Check sheet for the modelled part. Datum: model origin and axes. Units: mm. A direction names the side the tool comes from. Round coordinates to 2 decimals unless told otherwise and drop trailing zeros. Order: outer loops, then holes, each group sorted by start corner. A loop starts at its lowest first (then second) coordinate and runs counter-clockwise, first axis right, second up.
(1) Sectioned sample at B-B, the plane z = 25. Enter the section's corners in (x, y), and give its area (3 significant figures).
(2) Sectioned sample at A-A, the plane z = 10. Enter the section's corners in (x, y).
(3) Sectioned sample at C-C, the plane y = -3.5. Enter the section's corners in (x, z), and give its area (3 significant figures).
(4) Tool access check on faces 5 (the flat face through (3, -20, 2)), 6 (the flat face through (0, 6.716, 13)), 7 (the cylindrical face through (1.739, -15.325, 13.205)), 8 (the cylindrical face through (2.314, -14.176, 20.762)). Record the directions out of +Z, -Z, +X, -X, +Y, -Y that give a thin tool (end or side, any length) a straight path to the whole face; none if there is none.
(5) Depth check by flat-ended pin: pin 1 (3.5 mm diameter, centred on x = -11, y = -21.5, fed in from +Z); pin 2 (3 mm diameter, centred on x = -11, z = 14.5, fed in from -Y); pin 3 (1.4 mm diameter, centred on y = 7.5, z = 11.5, fed in from +X). Enter the tip coordinate at first touch or a pass-through.
(6) Thickness scan on probe 1 along Y at (x, z) = (11.5, 13); probe 2 along Z at (x, y) = (0.5, -11.5); probe 3 along Y at (x, z) = (23, 18.5). Record the ranges inside material, lowest first.
(7) Mould release check, pull along Y, two halves, no side actions. Record for faces 1 (the flat face through (2, -6, 2)), 2 (the flat face through (22.89, -6.12, 1.01)), 3 (the cylindrical face through (-2.361, -18.603, 8.761)), 4 (the flat face through (18, -21, 2)): released by +Y, released by -Y, zero draft, split by the parting line, or undercut.
```python
from build123d import *

# Parameters (mm, degrees)
CROQUIS1_W              = 60
CROQUIS1_H              = 30
SALIENTE_EXTRUIR1_DEPTH = 2
SALIENTE_EXTRUIR2_DEPTH = 38
SALIENTE_EXTRUIR4_DEPTH = 2
REDONDEO1_R             = 2
REDONDEO2_R             = 1
CORTAR_EXTRUIR2_DEPTH   = 2
CROQUIS7_W              = 20
CROQUIS7_H              = 20
SALIENTE_EXTRUIR5_DEPTH = 2.7
CROQUIS8_R              = 1.75
CORTAR_EXTRUIR3_DEPTH   = 2.7
CROQUIS11_R             = 3.36
CORTAR_EXTRUIR4_DEPTH   = 50
SALIENTE_EXTRUIR3_DEPTH = 15
CORTAR_EXTRUIR1_START   = -12.5
CORTAR_EXTRUIR1_DEPTH   = 12.5


with BuildPart() as part:
    # Croquis1 → Saliente-Extruir1 (new body)
    with BuildSketch(Plane.XY):
        with Locations((2.747988453, -8.28358209)):
            Rectangle(CROQUIS1_W, CROQUIS1_H)
    extrude(amount=SALIENTE_EXTRUIR1_DEPTH)

    # Croquis2 → Saliente-Extruir2 (add)
    with BuildSketch(Plane.XY.offset(2)):
        with BuildLine():
            Line((-27.252011547, -23.28358209), (-27.252011547, -20.794473938))
            ThreePointArc((-27.252011547, -20.794473938), (2.747988453, -14.174360447), (32.747988453, -20.794473938))
            Line((32.747988453, -20.794473938), (32.747988453, -23.28358209))
            ThreePointArc((32.747988453, -23.28358209), (2.747988453, -16.424360447), (-27.252011547, -23.28358209))
        make_face()
    extrude(amount=SALIENTE_EXTRUIR2_DEPTH)

    # Croquis5 → Saliente-Extruir4 (add)
    with BuildSketch(Plane.XY.offset(40)):
        with BuildLine():
            Line((32.747988453, -23.28358209), (32.747988453, -18.596159377))
            ThreePointArc((32.747988453, -18.596159377), (2.747988453, -12.174360447), (-27.252011547, -18.596159377))
            Line((-27.252011547, -18.596159377), (-27.252011547, -23.28358209))
            ThreePointArc((-27.252011547, -23.28358209), (2.747988453, -16.424360447), (32.747988453, -23.28358209))
        make_face()
    extrude(amount=SALIENTE_EXTRUIR4_DEPTH)

    # Redondeo1
    redondeo1_edges = [part.edges().sort_by_distance(p)[0] for p in [
        (2.747988453, -14.174360447, 2),
        (2.747988453, -14.174360447, 40),
    ]]
    fillet(redondeo1_edges, radius=REDONDEO1_R - 0.0001)  # a hair under: the kernel refuses the full size

    # Redondeo2
    redondeo2_edges = [part.edges().sort_by_distance(p)[0] for p in [
        (2.747988453, -12.174360447, 40),
    ]]
    fillet(redondeo2_edges, radius=REDONDEO2_R)

    # Croquis6 → Cortar-Extruir2 (cut)
    with BuildSketch(Plane.XY.offset(2)):
        Polygon((-27.252011547, -18.596159377), (-7.252011547, 6.71641791), (-27.252011547, 6.71641791), align=None)
        Polygon((12.747988453, 6.71641791), (32.747988453, 6.71641791), (32.747988453, -18.596159377), align=None)
    extrude(amount=-CORTAR_EXTRUIR2_DEPTH, mode=Mode.SUBTRACT)

    # Croquis7 → Saliente-Extruir5 (add)
    with BuildSketch(Plane(origin=(0, 6.71641791, 0), x_dir=(1, 0, 0), z_dir=(0, 1, 0))):
        with Locations((2.747988453, -10)):
            Rectangle(CROQUIS7_W, CROQUIS7_H)
    extrude(amount=SALIENTE_EXTRUIR5_DEPTH)

    # Croquis8 → Cortar-Extruir3 (cut)
    with BuildSketch(Plane(origin=(0, 9.41641791, 0), x_dir=(1, 0, 0), z_dir=(0, 1, 0))):
        with Locations(Location((2.747988453, -10, 0), (0, 0, 270))):
            Circle(CROQUIS8_R)
    extrude(amount=-CORTAR_EXTRUIR3_DEPTH, mode=Mode.SUBTRACT)

    # Croquis10 → Refrentado para tornillo tapón con cabeza plana de clavija de M31 (revolve, cut)
    with BuildSketch(Plane(origin=(2.747988453, 6.71641791, 10), x_dir=(0, 0, -1), z_dir=(1, 0, 0))):
        Polygon((0, 0), (0, 2.7), (1.7, 2.7), (1.7, 1.66), (3.36, 0), align=None)
    revolve(axis=Axis((2.747988453, 0.36641791, 10), (0, 1, 0)), mode=Mode.SUBTRACT)

    # Croquis11 → Cortar-Extruir4 (cut)
    with BuildSketch(Plane.XZ.offset(-6.71641791)):
        with Locations(Location((2.747988453, 10, 0), (0, 0, 90))):
            Circle(CROQUIS11_R)
    extrude(amount=CORTAR_EXTRUIR4_DEPTH, mode=Mode.SUBTRACT)

    # Croquis3 → Saliente-Extruir3 (add)
    with BuildSketch(Plane.XY.offset(2)):
        with BuildLine():
            Line((-1.252011547, -23.28358209), (-1.252011547, -16.540341587))
            ThreePointArc((-1.252011547, -16.540341587), (-2.377695965, -16.614909121), (-3.502011547, -16.70786179))
            Line((-3.502011547, -16.70786179), (-3.502011547, -23.28358209))
            Line((-3.502011547, -23.28358209), (-1.252011547, -23.28358209))
        make_face()
        with BuildLine():
            Line((8.997988453, -23.28358209), (8.997988453, -16.70786179))
            ThreePointArc((8.997988453, -16.70786179), (7.873672871, -16.614909121), (6.747988453, -16.540341587))
            Line((6.747988453, -16.540341587), (6.747988453, -23.28358209))
            Line((6.747988453, -23.28358209), (8.997988453, -23.28358209))
        make_face()
    extrude(amount=SALIENTE_EXTRUIR3_DEPTH)

    # Croquis4 → Cortar-Extruir1 (cut)
    with BuildSketch(Plane.ZY.offset(3.502011547).offset(CORTAR_EXTRUIR1_START)):
        with BuildLine():
            Line((17, -16.70786179), (17, -23.28358209))
            Line((17, -23.28358209), (2, -23.28358209))
            ThreePointArc((2, -23.28358209), (8.868759287, -18.555786805), (17, -16.70786179))
        make_face()
    extrude(amount=CORTAR_EXTRUIR1_DEPTH, mode=Mode.SUBTRACT)


solid = part.part
```
Derived:
1. outline: (-27.25, -23.28) arc R69.03 cw to (32.75, -23.28) - (32.75, -20.79) arc R71.28 ccw to (-27.25, -20.79) - close
1. area: 139 mm2
2. outline: (-27.25, -23.28) arc R69.03 cw to (-3.5, -16.71) - (-3.5, -18.1) - (-1.25, -18.1) - (-1.25, -16.54) arc R69.03 cw to (-0.61, -16.51) - (-0.61, -14.25) arc R71.28 ccw to (-27.25, -20.79) - close; (-7.25, 6.72) - (-0.61, 6.72) - (1, 8.33) - (1, 9.42) - (-7.25, 9.42) - close; (4.5, 8.33) - (6.11, 6.72) - (12.75, 6.72) - (12.75, 9.42) - (4.5, 9.42) - close; (6.11, -16.51) arc R69.03 cw to (6.75, -16.54) - (6.75, -18.1) - (9, -18.1) - (9, -16.71) arc R69.03 cw to (32.75, -23.28) - (32.75, -20.79) arc R71.28 ccw to (6.11, -14.25) - close
3. outline: (-15.32, 0) - (20.82, 0) - (20.82, 2) - (-15.32, 2) - close
3. area: 72.3 mm2
4. face 5: +Z, -Y
4. face 6: +Z, +X, -X
4. face 7: -Y
4. face 8: none
5. pin 1: stops at z = 2
5. pin 2: stops at y = -18.13
5. pin 3: stops at x = 12.75
6. probe 1: y = -16.98 to -14.71, 6.72 to 9.42
6. probe 2: z = 0 to 2
6. probe 3: y = -19.46 to -17.11
7. face 1: undercut
7. face 2: released by +Y
7. face 3: released by -Y
7. face 4: zero draft
